Geometry: see drawing. Coordinates: mm, zero at the bounding-box minimum. A direction names the side the tool comes from. Coordinates: 2 decimals unless noted, no trailing zeros. Write each loop counter-clockwise with the first axis right and the second up, starting at its lowest first coordinate (ties: lowest second). Pieces come first, ordered by that corner, then holes. Notation, with made-up numbers: M -4.75,-39.75 L 3.25,-39.75 A12 ccw 3.25,-35.75 Z; hole C -14,86 d4. An arc over 180 degrees is marked long. Answer as CSV lines item,"result". Start each with the question number.
1. Reachability of the marked faces 1, 2 and 3 from +Z, -Z, +X, -X, +Y, -Y: full face, straight path, thin tool, end or side. Return the list, or none.
2. Section D-D on z = 20.5. Return the cut outline in (x, y).
3. Contact query for flat-ended pins moving along their axis: pin 1 Ø2 at (y, z) = (5, 11.5) entering from -X; pin 2 Ø2 at (y, z) = (3.5, 18) entering from +X; pin 3 Ø1.5 at (x, y) = (13, 5) entering from +Z. Output: stop coordinate, or through.
4. Section A-A on z = 11.5. Return the cut outline in (x, y).
5. Section C-C on y = 0.5. Return the cut outline in (x, z), plus the area to 3 significant figures.
6. Section B-B on x = 12.95. Return the cut outline in (y, z).
7. Mould query, pull axis Z, two halves, no side actions, for the marked faces 4, 5 and 6. Classes: pulls with the +Z half, pulls with the -Z half, needs draft (parallel to the pull), parting line crosses it, or undercut.
8. Line query: probe 1 along X at (y, z) = (3.7, 11.5); probe 2 along X at (y, z) = (1.65, 11.5); probe 3 along Z at (x, y) = (10.75, 4.75). Output: solid intervals per line, ascending. Write a range as [from, to].
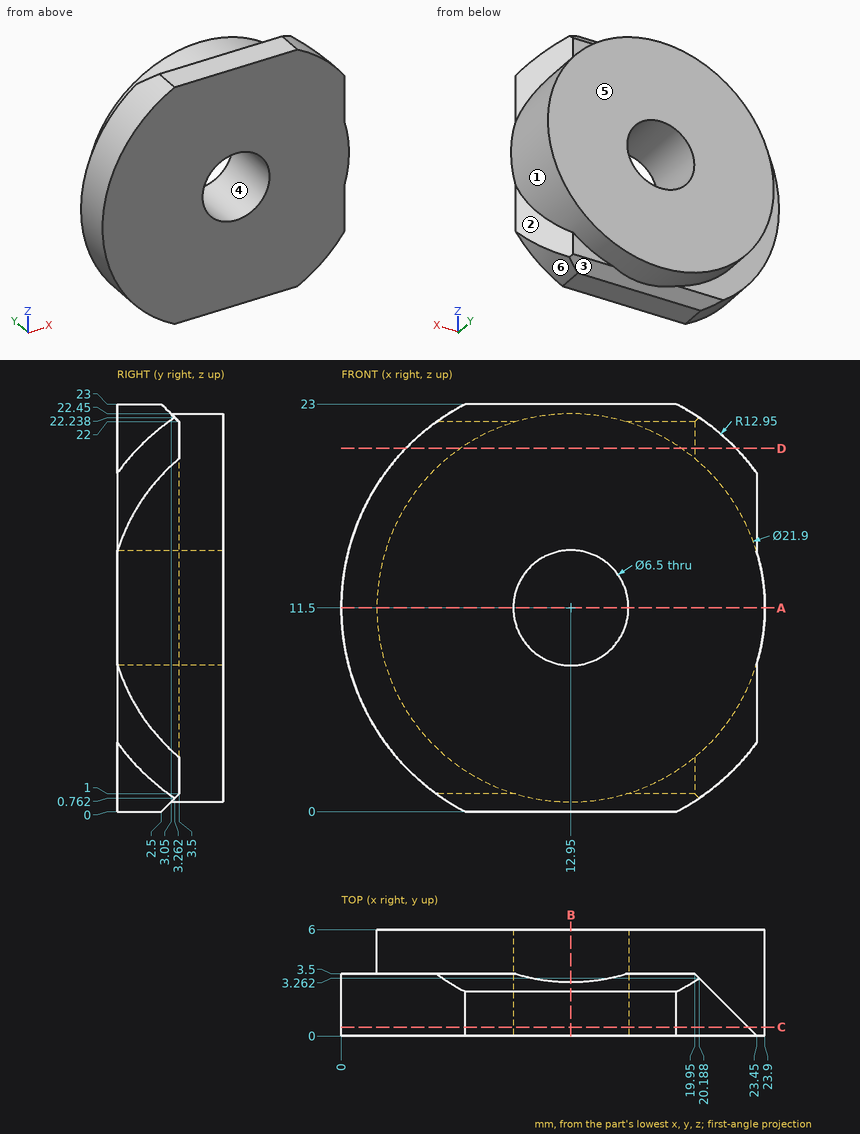
Values:
1,face 1,"+Y"
1,face 2,"-Z, +X, +Y"
1,face 3,"-Z, +Y"
2,outline,"M 3.64,0 L 22.26,0 L 22.26,1.19 L 19.95,3.5 L 19.19,3.5 L 19.19,6 L 6.71,6 L 6.71,3.5 L 3.64,3.5 Z"
3,pin 1,"x = 2"
3,pin 2,"x = 22.42"
3,pin 3,"z = 22.45"
4,outline,"M 0,0 L 9.7,0 L 9.7,6 L 2,6 L 2,3.5 L 0,3.5 Z; M 16.2,0 L 23.9,0 L 23.9,6 L 16.2,6 Z"
5,outline,"M 7,0 L 18.9,0 A12.95 ccw 22.95,3.27 L 22.95,7.04 A10.95 ccw 22.95,15.96 L 22.95,19.73 A12.95 ccw 18.9,23 L 7,23 A12.95 ccw Z; hole C 12.95,11.5 d6.5"
5,area,"443 mm²"
6,outline,"M 0,0 L 2.5,0 L 3.05,0.55 L 6,0.55 L 6,8.25 L 0,8.25 Z; M 0,14.75 L 6,14.75 L 6,22.45 L 3.05,22.45 L 2.5,23 L 0,23 Z"
7,face 4,"undercut"
7,face 5,"needs draft"
7,face 6,"pulls with the -Z half"
8,probe 1,"[2, 9.7], [16.2, 23.9]"
8,probe 2,"[0, 9.7], [16.2, 23.9]"
8,probe 3,"[0.77, 9.11], [13.89, 22.23]"
